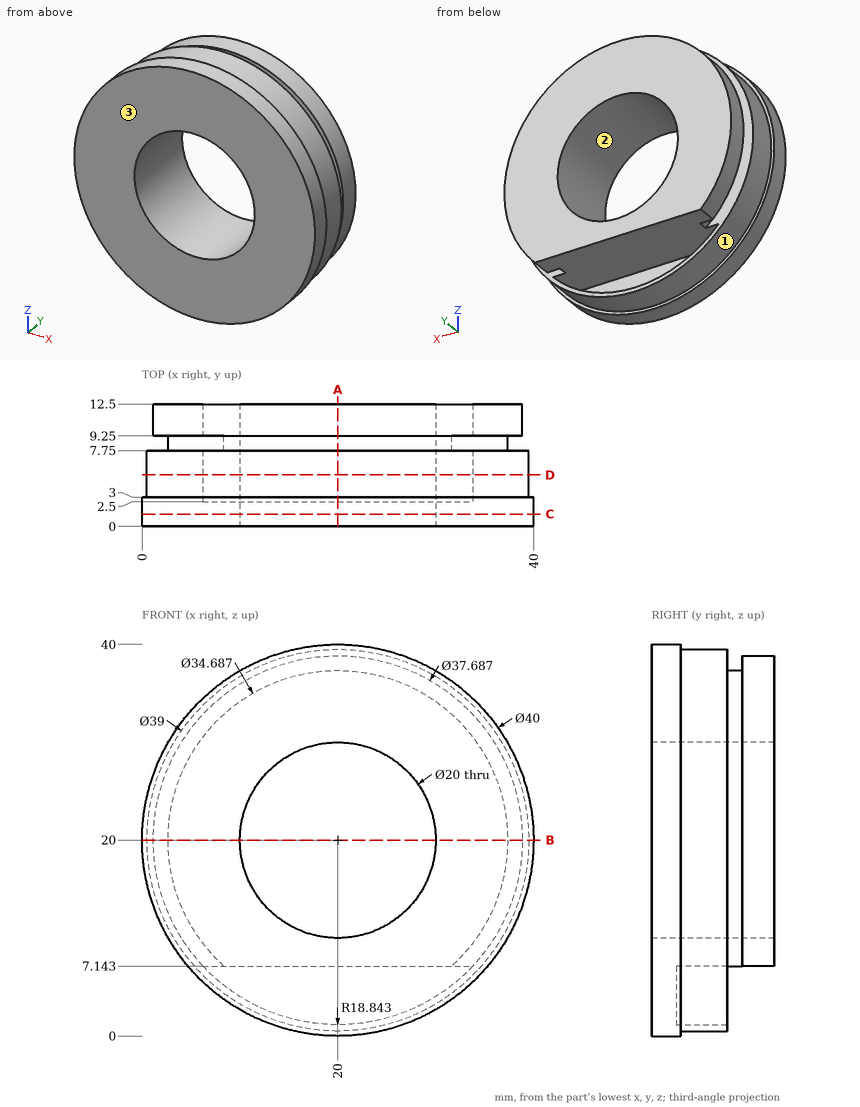
Design review of the part shown in the three views and the two pictorial views. Dimensions are in mm from the part's minimum x, y and z. Round coordinates to 2 decimals unless told otherwise and drop trailing zeros. Write each loop counter-clockwise with the first axis right and the second up, starting at its lowest first coordinate (ties: lowest second). Pieces come first, ordered by that corner, then holes. Notation, with made-up numbers: M -15.5,51 L 14.5,51 A15 ccw 14.5,60 Z; hole C 32,77 d1. An arc over 180 degrees is marked long. One line per item, written item: value. Start each with the question number.
1. Clearance check with flat-ended pins moving along their axes: P1, Ø3, axis at y = 11, z = 23, coming from the -X side; P2, Ø3, axis at x = 23.5, y = 8.5, coming from the -Z side (1 decimal); P3, Ø4, axis at y = 5, z = 12, coming from the -X side; P4, Ø12, axis at x = 22, z = 4.5, coming from the +Y side. State where each tip first meets the part, or that it passes through.
2. To check wall thickness, follow probe 1 along X at (y, z) = (3.5, 20); probe 2 along Z at (x, y) = (27, 7.25) (1 decimal); probe 3 along X at (y, z) = (9.75, 20). State the ranges of each line that lie inside material, in increasing order. Write a range as from..to.
3. Take a section at D-D on y = 5.25. State the section outline as (x, z) points.
4. Draft analysis for pull direction X (two halves, no side actions). For the marked faces 1, 2 and 3, state which applies: pulls with the +X half, pulls with the -X half, needs draft (parallel to the pull), parting line crosses it, or undercut.
5. Take a section at B-B on z = 20. State the section outline as (x, y) points, then the cut area to 3 significant figures.
6. Take a section at A-A on x = 20. State the section outline as (y, z) points, then the cut area to 3 significant figures.
7. Take a section at C-C on y = 1.25. State the section outline as (x, z) points.
Computed:
1. P1: stops at x = 1.22
1. P2: stops at z = 0.6
1. P3: stops at x = 1.45
1. P4: stops at y = 12.5
2. probe 1: x = 0.5..10, 30..39.5
2. probe 2: z = 1.8..2.5, 7.1..12.9, 27.1..38.2
2. probe 3: x = 1.16..10, 30..38.84
3. outline: C 20,20 d39; hole M 6.22,7.14 A18.84 ccw 33.78,7.14 Z; hole C 20,20 d20
4. face 1: parting line crosses it
4. face 2: undercut
4. face 3: needs draft
5. outline: M 0,0 L 10,0 L 10,12.5 L 1.16,12.5 L 1.16,9.25 L 2.66,9.25 L 2.66,7.75 L 0.5,7.75 L 0.5,3 L 0,3 Z; M 30,0 L 40,0 L 40,3 L 39.5,3 L 39.5,7.75 L 37.34,7.75 L 37.34,9.25 L 38.84,9.25 L 38.84,12.5 L 30,12.5 Z
5. area: 230 mm²
6. outline: M 0,0 L 3,0 L 3,0.5 L 7.75,0.5 L 7.75,1.16 L 2.5,1.16 L 2.5,7.14 L 12.5,7.14 L 12.5,10 L 0,10 Z; M 0,30 L 12.5,30 L 12.5,38.84 L 9.25,38.84 L 9.25,37.34 L 7.75,37.34 L 7.75,39.5 L 3,39.5 L 3,40 L 0,40 Z
6. area: 172 mm²
7. outline: C 20,20 d40; hole C 20,20 d20
